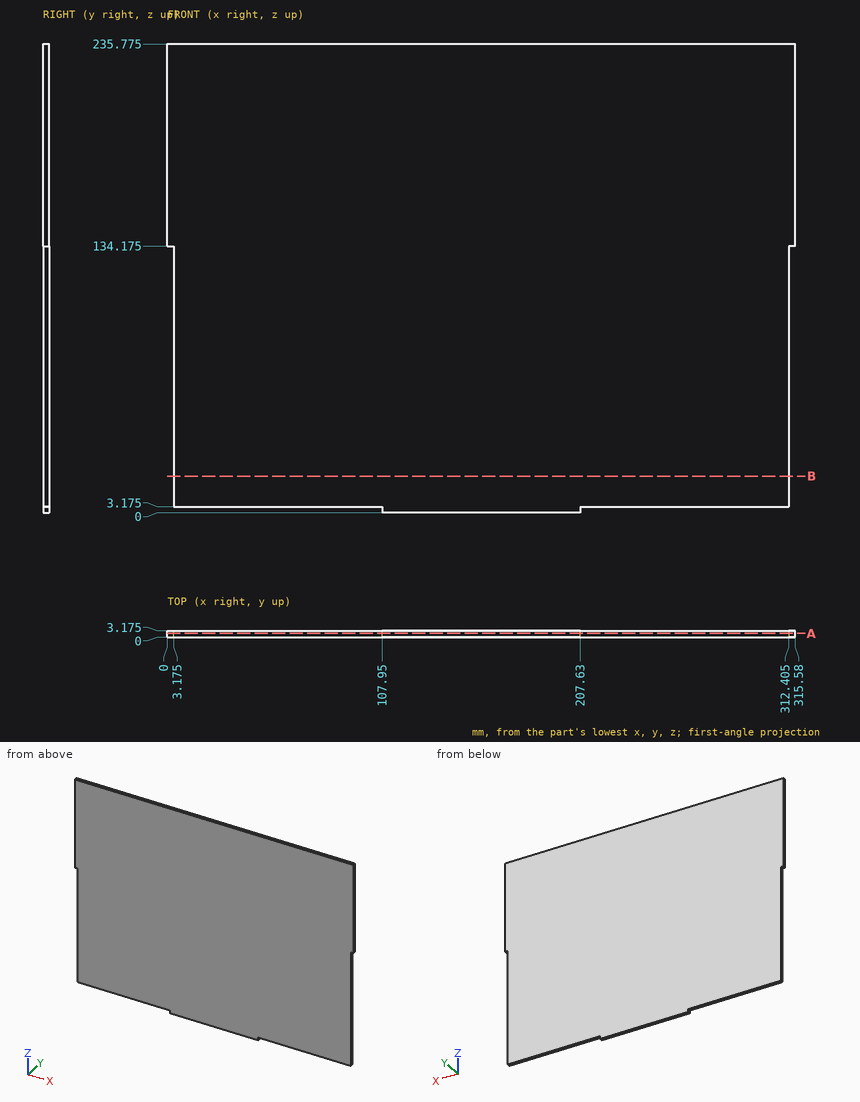
Part print with two shaded views. Sizes in mm from the minimum x, y, z corner. Give positions to 0.01 mm unless a question says otherwise; leave off trailing zeros. Order: outer loops, then holes, each group sorted by start corner. A loop starts at its lowest first (then second) coordinate and runs counter-clockwise, first axis right, second up.
1) Saw through at B-B, the plane z = 18.5. Write the cut outline in (x, y) (3 decimals), then the cut area to 3 significant figures.
2) Saw through at A-A, the plane y = 1.9. Write the cut outline in (x, z) (3 decimals).
3) Wall check: probe 1 along Z at (x, y) = (250, 1.1) (3 decimals); probe 2 along X at (y, z) = (1.6, 48.5) (3 decimals). Give the ranges that are in metal, low to high.
4) Pin check, flat tips, straight feed: pin 1 (1 mm diameter, centred on y = 1, z = 45, fed in from +X) (3 decimals); pin 2 (1 mm diameter, centred on y = 1, z = 75, fed in from -X) (3 decimals); pin 3 (1.6 mm diameter, centred on x = 1, y = 1, fed in from -Z) (3 decimals). Stop position of each tip, or through.
Computed:
1. outline: (3.175, 0) - (312.405, 0) - (312.405, 3.175) - (3.175, 3.175) - close
1. area: 982 mm2
2. outline: (0, 134.175) - (3.175, 134.175) - (3.175, 3.175) - (107.95, 3.175) - (107.95, 0) - (207.63, 0) - (207.63, 3.175) - (312.405, 3.175) - (312.405, 134.175) - (315.58, 134.175) - (315.58, 235.775) - (0, 235.775) - close
3. probe 1: z = 3.175 to 235.775
3. probe 2: x = 3.175 to 312.405
4. pin 1: stops at x = 312.405
4. pin 2: stops at x = 3.175
4. pin 3: stops at z = 134.175
